```python
from build123d import *

# Parameters (mm, degrees)
ENL_V_MAT_EXTRU_1_DEPTH      = 19
ENL_V_MAT_EXTRU_1_DEPTH_BACK = 19
ESQUISSE4_OUTSIDE_W          = 55.312
ESQUISSE4_OUTSIDE_H          = 55.312
ENL_V_MAT_EXTRU_2_DEPTH      = 10
ESQUISSE5_R                  = 4.5
BOSS_EXTRU_1_DEPTH           = 9
CHANFREIN1_SIZE              = 0.5


with BuildPart() as part:
    # Esquisse2 → Révolution2 (revolve)
    with BuildSketch(Plane(origin=(0, 0, 0), x_dir=(0, 0, -1), z_dir=(1, 0, 0))):
        Polygon((-36, 0), (-70, 0), (-70, 6), (-52, 6), (-52, 10), (-7, 10), (-7, 9), (-4, 9), (-4, 18), (0, 18), (0, 7), (-32, 7), align=None)
    revolve(axis=Axis((0, 0, 0), (0, 0, 1)))

    # Esquisse3 → Enlèv. mat.-Extru.1 (cut, two sides)
    with BuildSketch(Plane(origin=(0, 0, 0), x_dir=(0, 0, -1), z_dir=(1, 0, 0))) as enl_v_mat_extru_1_sk:
        with BuildLine():
            Line((-16, 10), (-28, 10))
            Line((-28, 10), (-28, 6))
            ThreePointArc((-28, 6), (-27.414213562, 4.585786438), (-26, 4))
            Line((-26, 4), (-18, 4))
            ThreePointArc((-18, 4), (-16.585786438, 4.585786438), (-16, 6))
            Line((-16, 6), (-16, 10))
        make_face()
    extrude(amount=ENL_V_MAT_EXTRU_1_DEPTH, mode=Mode.SUBTRACT)
    extrude(enl_v_mat_extru_1_sk.sketch, amount=-ENL_V_MAT_EXTRU_1_DEPTH_BACK, mode=Mode.SUBTRACT)

    # Esquisse4 outside → Enlèv. mat.-Extru.2 (cut)
    with BuildSketch(Plane(origin=(0, 0, 0), x_dir=(-1, 0, 0), z_dir=(0, 0, -1))):
        Rectangle(ESQUISSE4_OUTSIDE_W, ESQUISSE4_OUTSIDE_H)
        with BuildLine():
            Line((-18, 0), (-12, 0))
            Line((-12, 0), (-7, 16.583123952))
            ThreePointArc((-7, 16.583123952), (0, 18), (7, 16.583123952))
            Line((7, 16.583123952), (12, 0))
            Line((12, 0), (18, 0))
            ThreePointArc((18, 0), (0, -18), (-18, 0))
        make_face(mode=Mode.SUBTRACT)
    extrude(amount=-ENL_V_MAT_EXTRU_2_DEPTH, mode=Mode.SUBTRACT)

    # Esquisse5 → Boss.-Extru.1 (add)
    with BuildSketch(Plane(origin=(0, 0, 0), x_dir=(-1, 0, 0), z_dir=(0, 0, -1))):
        with Locations((0, 12.5)):
            Circle(ESQUISSE5_R)
    extrude(amount=BOSS_EXTRU_1_DEPTH)

    # Chanfrein1
    chanfrein1_edges = [part.edges().sort_by_distance(p)[0] for p in [
        (4.5, 12.5, 0),
        (0, -6, 70),
        (0, -18, 0),
    ]]
    chamfer(chanfrein1_edges, length=CHANFREIN1_SIZE)


solid = part.part
```
Read the model definition and answer for the solid it produces. Units are mm, in the model's axes. A direction names the side the tool comes from. Round coordinates to 2 decimals unless told otherwise and drop trailing zeros. Write each loop counter-clockwise with the first axis right and the second up, starting at its lowest first coordinate (ties: lowest second). Pieces come first, ordered by that corner, then holes. Notation, with made-up numbers: (51.5, 84) - (63.5, 84) arc R17 cw to (63.5, 111) - close; hole circle Ø1 at (20.5, 68). An arc over 180 degrees is marked (long way). One line per item, written item: value.
Q1. Which of the six approach directions +Z, -Z, +X, -X, +Y, -Y give full straight-line access (tool end or side, diameter ignored) to faces 4 (the flat face through (0, 13, -9)), 5 (the flat face through (0, 8, 28)), 6 (the cylindrical face through (0, -10, 29)), 7 (the flat face through (0, 0, 70)), 8 (the cylindrical face through (-2.419, 16.294, -4.69))?
The answers:
face 4: -Z, +X, -X, +Y, -Y
face 5: +X, -X, +Y
face 6: +Z
face 7: +Z, +X, -X, +Y, -Y
face 8: -Z
Q2. Straight lines are drawn through the part: line 1 (Z direction, x = 2, y = 7); line 2 (X direction, y = 0, z = 25). For each, find the intervals that lie inside material, in ascending order. Write a range as from..to.
The answers:
line 1: z = 0..16, 28..52
line 2: x = -10..-7, 7..10
Q3. Find section B-B (z = 62). Determine the outline of the cut face in (x, y), and give its area (3 significant figures).
The answers:
outline: circle Ø12 at (0, 0)
area: 113 mm2
Q4. For a pull along X with two mould halves and no side action, classify faces 1 (the cylindrical face through (6.96, 4.57, 16.6)), 2 (the cylindrical face through (0, -7, 16)), 3 (the cylindrical face through (0, -6, 61)) as pulls with the +X half, pulls with the -X half, needs draft (parallel to the pull), parting line crosses it, or undercut.
The answers:
face 1: needs draft
face 2: undercut
face 3: parting line crosses it
Q5. Each of these flat-tipped pins is pushed along its axis until it touches: P1, Ø4, axis at y = 2, z = 50.5, coming from the +X side; P2, Ø6, axis at x = 11.5, z = 23.5, coming from the +Y side; P3, Ø1.2, axis at x = -2, y = 7, coming from the +Z side. Where does it stop, or does it pass through?
The answers:
P1: stops at x = 10
P2: stops at y = 4
P3: stops at z = 52
Q6. Find section A-A (y = 12.5). Determine the outline of the cut face in (x, z).
The answers:
outline: (-8.23, 0) - (-5, 0) - (-4.5, -0.5) - (-4.5, -9) - (4.5, -9) - (4.5, -0.5) - (5, 0) - (8.23, 0) - (8.23, 4) - (-8.23, 4) - close
